Build history of the part. All positions in model axes, mm. Face numbers are marked on the shaded views. A direction names the side the tool comes from. Round coordinates to 2 decimals unless told otherwise and drop trailing zeros. Order: outer loops, then holes, each group sorted by start corner. A loop starts at its lowest first (then second) coordinate and runs counter-clockwise, first axis right, second up. Notation, with made-up numbers: (73.5, -25) -> (121.5, -25) arc R34 cw to (121.5, 9) -> close; hole circle Ø6 at (89.25, 75.25). An arc over 180 degrees is marked (long way). Answer as a JSON object with one key per item and string values.
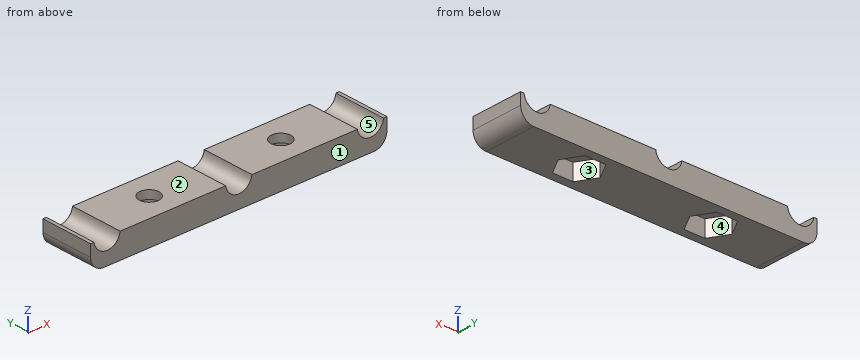
from build123d import *

# Parameters (mm, degrees)
BOSS_EXTRU_1_DEPTH      = 4
CONG_1_R                = 2
ESQUISSE2_R             = 1.5
ENL_V_MAT_EXTRU_1_DEPTH = 24.158421794
ENL_V_MAT_EXTRU_2_DEPTH = 2.5


with BuildPart() as part:
    # Esquisse1 → Boss.-Extru.1 (new, symmetric)
    with BuildSketch(Plane(origin=(0, 0, 0), x_dir=(1, 0, 0), z_dir=(0, 1, 0))):
        with BuildLine():
            Line((22.5, 4), (-22.5, 4))
            Line((-22.5, 4), (-22.5, 0.25))
            Line((-22.5, 0.25), (-21.984313483, 0.25))
            ThreePointArc((-21.984313483, 0.25), (-20, 2), (-18.015686517, 0.25))
            Line((-18.015686517, 0.25), (-1.984313483, 0.25))
            ThreePointArc((-1.984313483, 0.25), (0, 2), (1.984313483, 0.25))
            Line((1.984313483, 0.25), (18.015686517, 0.25))
            ThreePointArc((18.015686517, 0.25), (20, 2), (21.984313483, 0.25))
            Line((21.984313483, 0.25), (22.5, 0.25))
            Line((22.5, 0.25), (22.5, 4))
        make_face()
    extrude(amount=BOSS_EXTRU_1_DEPTH, both=True)

    # Congé1
    cong_1_edges = [part.edges().sort_by_distance(p)[0] for p in [
        (-22.5, 0, -4),
        (22.5, 0, -4),
    ]]
    fillet(cong_1_edges, radius=CONG_1_R)

    # Esquisse2 → Enlèv. mat.-Extru.1 (cut, through all)
    with BuildSketch(Plane.XY.offset(-0.25)):
        with Locations((-10, 0)):
            Circle(ESQUISSE2_R)
        with Locations((10, 0)):
            Circle(ESQUISSE2_R)
    extrude(amount=-ENL_V_MAT_EXTRU_1_DEPTH, mode=Mode.SUBTRACT)

    # Esquisse3 → Enlèv. mat.-Extru.2 (cut)
    with BuildSketch(Plane(origin=(0, 0, -4), x_dir=(-1, 0, 0), z_dir=(0, 0, -1))):
        Polygon((-8.41228676, 2.75), (-11.58771324, 2.75), (-13.175426481, 0), (-11.58771324, -2.75), (-8.41228676, -2.75), (-6.824573519, 0), align=None)
        Polygon((11.58771324, 2.75), (8.41228676, 2.75), (6.824573519, 0), (8.41228676, -2.75), (11.58771324, -2.75), (13.175426481, 0), align=None)
    extrude(amount=-ENL_V_MAT_EXTRU_2_DEPTH, mode=Mode.SUBTRACT)


solid = part.part
1) Cut at A-A, the plane z = -0.9. Give the cut face in (x, y), plus the area to 3 significant figures.
Checked values:
{"outline": "(-22.5, -4) -> (-21.79, -4) -> (-21.79, 4) -> (-22.5, 4) -> close; (-18.21, -4) -> (-1.79, -4) -> (-1.79, 4) -> (-18.21, 4) -> close; (1.79, -4) -> (18.21, -4) -> (18.21, 4) -> (1.79, 4) -> close; (21.79, -4) -> (22.5, -4) -> (22.5, 4) -> (21.79, 4) -> close; hole circle Ø3 at (-10, 0); hole circle Ø3 at (10, 0)", "area": "260 mm²"}
2) Pull direction Y, two halves, no side cores. Call the marked faces 1, 2 and 3: pulls with the +Y half, pulls with the -Y half, needs draft (parallel to the pull), parting line crosses it, or undercut.
Checked values:
{"face 1": "pulls with the -Y half", "face 2": "needs draft", "face 3": "undercut"}
3) Which spindle directions (+Z, -Z, +X, -X, +Y, -Y) get a long thin tool onto all of the face, cutting with end or side? Do the marked faces 4 and 5. Say none if no direction does.
Checked values:
{"face 4": "-Z", "face 5": "+Z, +Y, -Y"}
4) Probe L1, parallel to Y at x = 10, z = -1.2; L2, parallel to X at y = 1, z = -3.5; L3, parallel to X at y = 1.25, z = -3.3. List the from-to ranges inside material, lowest first. Write a range as from..to.
Checked values:
{"L1": "y = -4..-1.5, 1.5..4", "L2": "x = -21.82..-12.6, -7.4..7.4, 12.6..21.82", "L3": "x = -22.02..-12.45, -7.55..7.55, 12.45..22.02"}
5) Cut at C-C, the plane y = -3.5. Give the cut face in (x, z).
Checked values:
{"outline": "(-22.5, -2) arc R2 ccw to (-20.5, -4) -> (20.5, -4) arc R2 ccw to (22.5, -2) -> (22.5, -0.25) -> (21.98, -0.25) arc R2 cw to (18.02, -0.25) -> (1.98, -0.25) arc R2 cw to (-1.98, -0.25) -> (-18.02, -0.25) arc R2 cw to (-21.98, -0.25) -> (-22.5, -0.25) -> close"}
6) Cut at D-D, the plane z = -3.3. Give the cut face in (x, y), plus the area to 3 significant figures.
Checked values:
{"outline": "(-22.02, -4) -> (22.02, -4) -> (22.02, 4) -> (-22.02, 4) -> close; hole (-13.18, 0) -> (-11.59, -2.75) -> (-8.41, -2.75) -> (-6.82, 0) -> (-8.41, 2.75) -> (-11.59, 2.75) -> close; hole (6.82, 0) -> (8.41, -2.75) -> (11.59, -2.75) -> (13.18, 0) -> (11.59, 2.75) -> (8.41, 2.75) -> close", "area": "300 mm²"}
7) Cut at B-B, the plane x = 10. Give the cut face in (y, z).
Checked values:
{"outline": "(-4, -4) -> (-2.75, -4) -> (-2.75, -1.5) -> (-1.5, -1.5) -> (-1.5, -0.25) -> (-4, -0.25) -> close; (1.5, -1.5) -> (2.75, -1.5) -> (2.75, -4) -> (4, -4) -> (4, -0.25) -> (1.5, -0.25) -> close"}
